Design review of the part built by this model. Coordinates are the model's own, in mm. Face numbers are marked on the shaded views. A direction names the side the tool comes from. Give positions to 0.01 mm unless a question says otherwise; leave off trailing zeros. Loops run counter-clockwise (first coordinate to the right, second up) from the corner with the lowest first, then second, coordinate; pieces in that order, holes last.
from build123d import *

# Parameters (mm, degrees)
SKETCH2_R                 = 22.50059
BOSS_EXTRUDE1_DEPTH       = 7.62
TAP_DRILL_FOR_6_32_TAP1_D = 2.7051


with BuildPart() as part:
    # Sketch2 → Boss-Extrude1 (new, symmetric)
    with BuildSketch(Plane.XY):
        with BuildLine():
            Line((-27.58059, 27.58059), (-27.58059, 10.16))
            Line((-27.58059, 10.16), (-42.82059, 10.16))
            Line((-42.82059, 10.16), (-42.82059, 0))
            Line((-42.82059, 0), (42.82059, 0))
            Line((42.82059, 0), (42.82059, 10.16))
            Line((42.82059, 10.16), (27.58059, 10.16))
            Line((27.58059, 10.16), (27.58059, 27.58059))
            ThreePointArc((27.58059, 27.58059), (0, 55.16118), (-27.58059, 27.58059))
        make_face()
        with Locations(Location((0, 27.58059, 0), (0, 0, 180))):
            Circle(SKETCH2_R, mode=Mode.SUBTRACT)
    extrude(amount=BOSS_EXTRUDE1_DEPTH, both=True)

    # Tap Drill for #6-32 Tap1 (through all)
    with Locations(Plane(origin=(0, 10.16, 0), x_dir=(1, 0, 0), z_dir=(0, 1, 0))):
        with Locations((-38.75659, -3.556), (-31.64459, 3.556), (31.64459, 3.556), (38.75659, -3.556)):
            Hole(TAP_DRILL_FOR_6_32_TAP1_D / 2)


solid = part.part
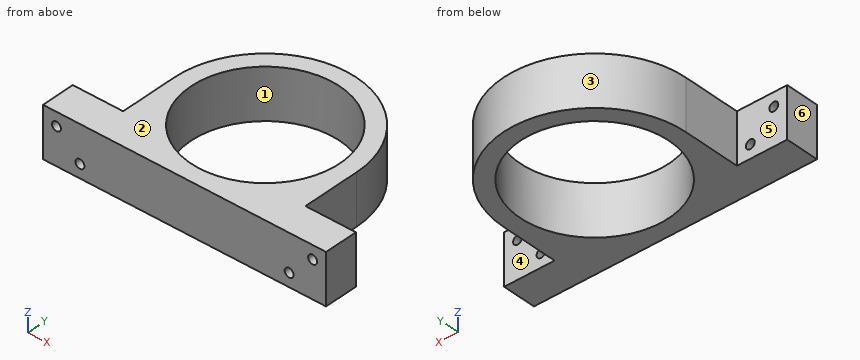
Q1. Wall thickness on line 1 (Y direction, x = 0, z = 3.5); line 2 (Y direction, x = -38.5, z = 6.5); line 3 (X direction, y = 21, z = 7.25): over which ranges is each line inside the solid? List them lowest first.
Results:
line 1: y = 0 to 5.08, 50.08 to 55.16
line 2: y = 0 to 10.16
line 3: x = -27.58 to -21.52, 21.52 to 27.58
Q2. Take a section at C-C (y = 18). Give the boundary of the cut face in (x, z).
Results:
outline: (-27.58, -7.62) - (-20.36, -7.62) - (-20.36, 7.62) - (-27.58, 7.62) - close; (20.36, -7.62) - (27.58, -7.62) - (27.58, 7.62) - (20.36, 7.62) - close
Q3. Take a section at B-B (x = 0). Give the boundary of the cut face in (y, z), plus the area to 3 significant figures.
Results:
outline: (0, -7.62) - (5.08, -7.62) - (5.08, 7.62) - (0, 7.62) - close; (50.08, -7.62) - (55.16, -7.62) - (55.16, 7.62) - (50.08, 7.62) - close
area: 155 mm2
Q4. Take a section at A-A (z = 6). Give the boundary of the cut face in (x, y), plus the area to 3 significant figures.
Results:
outline: (-42.82, 0) - (42.82, 0) - (42.82, 10.16) - (27.58, 10.16) - (27.58, 27.58) arc R27.58 ccw to (-27.58, 27.58) - (-27.58, 10.16) - (-42.82, 10.16) - close; hole circle Ø45 at (0, 27.58)
area: 1,440 mm2
Q5. Insertion check: pin 1 (8 mm diameter, centred on x = -2, z = -5, fed in from +Y); pin 2 (4 mm diameter, centred on x = 19.5, z = -3.5, fed in from +Y); pin 3 (4 mm diameter, centred on y = 12.5, z = 3.5, fed in from +X). Each pin has a flat end and moves straight along its axis. Give the tip position at first contact, or say it passes through.
Results:
pin 1: stops at y = 55.16
pin 2: stops at y = 48.9
pin 3: stops at x = 27.58
Q6. Take a section at D-D (x = 35). Give the boundary of the cut face in (y, z), plus the area to 3 significant figures.
Results:
outline: (0, -7.62) - (10.16, -7.62) - (10.16, 7.62) - (0, 7.62) - close
area: 155 mm2
Q7. Tool access review of the marked faces 4, 5 and 6: name each direction out of +Z, -Z, +X, -X, +Y, -Y from which nothing blocks a thin tool from reaching the whole face with its end or side.
Results:
face 4: +Z, -Z, +X, +Y
face 5: +Z, -Z, -X, +Y
face 6: +Z, -Z, -X, +Y, -Y
Q8. Draft analysis for pull direction Y (two halves, no side actions). For the marked faces 1, 2 and 3, state which applies: pulls with the +Y half, pulls with the -Y half, needs draft (parallel to the pull), parting line crosses it, or undercut.
Results:
face 1: undercut
face 2: needs draft
face 3: pulls with the +Y half
